Geometry check sheet. Reference: the model listing, model coordinates, mm. A direction names the side the tool comes from. Round coordinates to 2 decimals unless told otherwise and drop trailing zeros. Loops run counter-clockwise (first coordinate to the right, second up) from the corner with the lowest first, then second, coordinate; pieces in that order, holes last.
```python
from build123d import *

# Parameters (mm, degrees)
SKETCH3_W           = 28
SKETCH3_H           = 50
BOSS_EXTRUDE1_DEPTH = 14
SKETCH6_R           = 12.5
CUT_EXTRUDE1_DEPTH  = 40


with BuildPart() as part:
    # Sketch3 → Boss-Extrude1 (new body, symmetric)
    with BuildSketch(Plane(origin=(0, 0, 0), x_dir=(0, 0, -1), z_dir=(1, 0, 0))):
        with Locations((14, 25)):
            Rectangle(SKETCH3_W, SKETCH3_H)
    extrude(amount=BOSS_EXTRUDE1_DEPTH, both=True)

    # Sketch6 → Cut-Extrude1 (cut)
    with BuildSketch(Plane(origin=(0, 0, 0), x_dir=(-1, 0, 0), z_dir=(0, -1, 0))):
        with Locations((0, 14)):
            Circle(SKETCH6_R)
    extrude(amount=-CUT_EXTRUDE1_DEPTH, mode=Mode.SUBTRACT)


solid = part.part
```
1) Access from +Z, -Z, +X, -X, +Y, -Y to the whole of each face (thin tool, end or side, straight path). Record for faces 4 (the face through (0, 0, -1)), 5 (the face through (2.71, 19.72, -1.797)).
Report:
face 4: +Z, -Z, +X, -X, -Y
face 5: -Y
2) Gauge pin test, flat end, axial feed: pin 1 (4 mm diameter, centred on x = -6, z = -10, fed in from -Y). Record the tip position at first contact, or that the pin passes through.
Report:
pin 1: stops at y = 40
3) Mould release check, pull along X, two halves, no side actions. Record for faces 1 (the face through (0, 40, -14)), 2 (the face through (-14, 25, -14)), 3 (the face through (0, 50, -14)): +X half, -X half, draft (parallel to the pull), parting line (faces both ways), or undercut.
Report:
face 1: undercut
face 2: -X half
face 3: draft
4) Sectioned sample at C-C, the plane x = 0. Record the cut outline in (y, z), then the cut area to 3 significant figures.
Report:
outline: (0, -28) - (50, -28) - (50, 0) - (0, 0) - (0, -1.5) - (40, -1.5) - (40, -26.5) - (0, -26.5) - close
area: 400 mm2
5) Sectioned sample at A-A, the plane z = -14. Record the cut outline in (x, y).
Report:
outline: (-14, 0) - (-12.5, 0) - (-12.5, 40) - (12.5, 40) - (12.5, 0) - (14, 0) - (14, 50) - (-14, 50) - close
6) Sectioned sample at B-B, the plane y = 22. Record the cut outline in (x, z), then the cut area to 3 significant figures.
Report:
outline: (-14, -28) - (14, -28) - (14, 0) - (-14, 0) - close; hole circle Ø25 at (0, -14)
area: 293 mm2
7) Scan lines: line 1 along Z through (x, y) = (0, 12); line 2 along X through (y, z) = (12.5, -14); line 3 along X through (y, z) = (32, -18). Record each from-to range of solid material in increasing order.
Report:
line 1: z = -28 to -26.5, -1.5 to 0
line 2: x = -14 to -12.5, 12.5 to 14
line 3: x = -14 to -11.84, 11.84 to 14
